```python
from build123d import *

# Parameters (mm, degrees)
BOSS_EXTRUDE1_DEPTH      = 2
BOSS_EXTRUDE2_DEPTH      = 15
BOSS_EXTRUDE2_DEPTH_BACK = 2
CUT_EXTRUDE1_DEPTH       = 15
CUT_EXTRUDE2_DEPTH       = 15
SKETCH5_R                = 1.5
CUT_EXTRUDE3_DEPTH       = 15
SKETCH6_R                = 1.5
CUT_EXTRUDE4_DEPTH       = 15
SKETCH7_R                = 1.5
CUT_EXTRUDE5_DEPTH       = 15


with BuildPart() as part:
    # Sketch1 → Boss-Extrude1 (new body)
    with BuildSketch(Plane(origin=(0, 0, 0), x_dir=(1, 0, 0), z_dir=(0, 1, 0))):
        Polygon((0, 15), (15, 0), (0, 0), align=None)
    extrude(amount=BOSS_EXTRUDE1_DEPTH)

    # Sketch2 → Boss-Extrude2 (add, two sides: drawn at the far end of the back side and taken through both)
    with BuildSketch(Plane(origin=(0, 2, 0), x_dir=(1, 0, 0), z_dir=(0, 1, 0)).offset(-BOSS_EXTRUDE2_DEPTH_BACK)):
        Polygon((-2, -2), (15, -2), (15, 0), (0, 0), (0, 15), (-2, 15), align=None)
    extrude(amount=BOSS_EXTRUDE2_DEPTH + BOSS_EXTRUDE2_DEPTH_BACK)

    # Sketch3 → Cut-Extrude1 (cut)
    with BuildSketch(Plane(origin=(0, 0, 0), x_dir=(0, 0, -1), z_dir=(1, 0, 0))):
        Polygon((15, 2), (0, 17), (15, 17), align=None)
    extrude(amount=-CUT_EXTRUDE1_DEPTH, mode=Mode.SUBTRACT)

    # Sketch4 → Cut-Extrude2 (cut)
    with BuildSketch(Plane(origin=(0, 0, 0), x_dir=(-1, 0, 0), z_dir=(0, 0, -1))):
        Polygon((0, 17), (-15, 2), (-15, 17), align=None)
    extrude(amount=-CUT_EXTRUDE2_DEPTH, mode=Mode.SUBTRACT)

    # Sketch5 → Cut-Extrude3 (cut)
    with BuildSketch(Plane(origin=(0, 0, 0), x_dir=(0, 0, -1), z_dir=(1, 0, 0))):
        with Locations((2.550252532, 10.207106781)):
            Circle(SKETCH5_R)
        with Locations((8.207106781, 4.550252532)):
            Circle(SKETCH5_R)
    extrude(amount=-CUT_EXTRUDE3_DEPTH, mode=Mode.SUBTRACT)

    # Sketch6 → Cut-Extrude4 (cut)
    with BuildSketch(Plane(origin=(0, 0, 0), x_dir=(-1, 0, 0), z_dir=(0, 0, -1))):
        with Locations((-2.550252532, 10.207106781)):
            Circle(SKETCH6_R)
        with Locations((-8.207106781, 4.550252532)):
            Circle(SKETCH6_R)
    extrude(amount=-CUT_EXTRUDE4_DEPTH, mode=Mode.SUBTRACT)

    # Sketch7 → Cut-Extrude5 (cut)
    with BuildSketch(Plane(origin=(0, 2, 0), x_dir=(1, 0, 0), z_dir=(0, 1, 0))):
        with Locations(Location((2.550252532, 8.207106781, 0), (0, 0, 270))):
            Circle(SKETCH7_R)
        with Locations(Location((8.207106781, 2.550252532, 0), (0, 0, 270))):
            Circle(SKETCH7_R)
    extrude(amount=-CUT_EXTRUDE5_DEPTH, mode=Mode.SUBTRACT)


solid = part.part
```
Part model, mm, in its own coordinate system. A direction names the side the tool comes from. Round coordinates to 2 decimals unless told otherwise and drop trailing zeros. Loops run counter-clockwise (first coordinate to the right, second up) from the corner with the lowest first, then second, coordinate; pieces in that order, holes last. Notation, with made-up numbers: (52, 77) -> (109, 77) arc R20 ccw to (109, 92) -> close; hole circle Ø10 at (83.25, 69). An arc over 180 degrees is marked (long way). Use CSV: the item, a comma, the result in double quotes. Start each with the question number.
1) Cut at C-C, the plane z = -11.75. Write the cut outline in (x, y).
2) Which spindle directions (+Z, -Z, +X, -X, +Y, -Y) get a long thin tool onto all of the face, cutting with end or side? Do faces 5 (the flat face through (4, 6, 0)), 6 (the flat face through (7, 1, -8)). Say none if no direction does.
3) Wall check: L1, parallel to Z at x = 4.75, y = 8.75; L2, parallel to X at y = 7.75, z = -2.75. Give the ranges that are in metal, low to high. Write a range as [from, to].
4) Pull direction X, two halves, no side cores. Call faces 1 (the cylindrical face through (2.875, 8.743, 0.986)), 2 (the flat face through (7, 10, 1)), 3 (the cylindrical face through (9.706, 4.616, 0.986)), 4 (the flat face through (4, 2, -4)): +X half, -X half, draft (parallel to the pull), parting line (faces both ways), or undercut.
5) Cut at B-B, the plane x = 11.25. Write the cut outline in (y, z), plus the area to 3 significant figures.
6) Cut at A-A, the plane y = 10.75. Write the cut outline in (x, z), plus the area to 3 significant figures.
7) Cut at D-D, the plane x = 3.25. Write the cut outline in (y, z).
8) Drop flat-ended pins along their axis: P1, Ø2.5, axis at x = 8.21, z = -2.55, coming from the +Y side; P2, Ø5, axis at y = 10.21, z = -2.55, coming from the +X side; P3, Ø8, axis at y = 2, z = -7, coming from the +X side; P4, Ø4, axis at x = 2.55, z = -8.21, coming from the +Y side. Give the stop position or say it passes through.
Determined:
1,outline,"(-2, 0) -> (3.25, 0) -> (3.25, 2) -> (0, 2) -> (0, 5.25) -> (-2, 5.25) -> close"
2,face 5,"-Z, +X, +Y"
2,face 6,"-Z, +X, +Y, -Y"
3,L1,"z = [0, 2]"
3,L2,"x = [-2, 0]"
4,face 1,"undercut"
4,face 2,"+X half"
4,face 3,"undercut"
4,face 4,"draft"
5,outline,"(0, -3.75) -> (2, -3.75) -> (2, 0) -> (5.75, 0) -> (5.75, 2) -> (0, 2) -> close"
5,area,"19.0 mm2"
6,outline,"(-2, -6.25) -> (0, -6.25) -> (0, -3.95) -> (-2, -3.95) -> close; (-2, -1.15) -> (0, -1.15) -> (0, 0) -> (1.15, 0) -> (1.15, 2) -> (-2, 2) -> close; (3.95, 0) -> (6.25, 0) -> (6.25, 2) -> (3.95, 2) -> close"
6,area,"17.8 mm2"
7,outline,"(0, -11.75) -> (2, -11.75) -> (2, -9.53) -> (0, -9.53) -> close; (0, -6.88) -> (2, -6.88) -> (2, 0) -> (8.88, 0) -> (8.88, 2) -> (0, 2) -> close; (11.53, 0) -> (13.75, 0) -> (13.75, 2) -> (11.53, 2) -> close"
8,P1,"passes through"
8,P2,"stops at x = 0"
8,P3,"stops at x = 12"
8,P4,"stops at y = 2"
